from build123d import *

# Parameters (mm, degrees)
SKETCH1_W                = 110
SKETCH1_H                = 80
BOSS_EXTRUDE1_DEPTH      = 7.5
SKETCH3_W                = 110
SKETCH3_H                = 8
BOSS_EXTRUDE2_DEPTH      = 12
BOSS_EXTRUDE2_DEPTH_BACK = 12


with BuildPart() as part:
    # Sketch1 → Boss-Extrude1 (new body)
    with BuildSketch(Plane.XY):
        with Locations((0, 40)):
            Rectangle(SKETCH1_W, SKETCH1_H)
        with BuildLine():
            ThreePointArc((-27.981, 50.8), (-42.49917604, 41.099264909), (-45.905621202, 58.224621202))
            Line((-45.905621202, 58.224621202), (-38.481, 65.649242405))
            Line((-38.481, 65.649242405), (-31.056378798, 58.224621202))
            ThreePointArc((-31.056378798, 58.224621202), (-28.780264909, 54.81817604), (-27.981, 50.8))
        make_face(mode=Mode.SUBTRACT)
        with BuildLine():
            ThreePointArc((27.981, 50.8), (28.780264909, 54.81817604), (31.056378798, 58.224621202))
            Line((31.056378798, 58.224621202), (38.481, 65.649242405))
            Line((38.481, 65.649242405), (45.905621202, 58.224621202))
            ThreePointArc((45.905621202, 58.224621202), (48.181735091, 54.81817604), (48.981, 50.8))
            ThreePointArc((48.981, 50.8), (38.481, 40.3), (27.981, 50.8))
        make_face(mode=Mode.SUBTRACT)
    extrude(amount=BOSS_EXTRUDE1_DEPTH)

    # Sketch3 → Boss-Extrude2 (add, two sides)
    with BuildSketch(Plane.XY.offset(7.5)) as boss_extrude2_sk:
        with Locations((0, 4)):
            Rectangle(SKETCH3_W, SKETCH3_H)
    extrude(amount=BOSS_EXTRUDE2_DEPTH)
    extrude(boss_extrude2_sk.sketch, amount=-BOSS_EXTRUDE2_DEPTH_BACK)


solid = part.part
Input: part model. Units: mm. Frame: model coordinates. A direction names the side the tool comes from. Coordinates: 2 decimals unless noted, no trailing zeros. Loops run counter-clockwise (first coordinate to the right, second up) from the corner with the lowest first, then second, coordinate; pieces in that order, holes last.
Q1. Cut plane A-A (x = -3). Output: boundary loops of the cut face in (y, z), then the cut area to 3 significant figures.
Q2. Contact query for flat-ended pins moving along their axis: pin 1 (10 mm diameter, centred on x = -17.5, y = 64, fed in from -Z); pin 2 (3 mm diameter, centred on x = 12, y = 13, fed in from +Z); pin 3 (1 mm diameter, centred on x = 17.5, z = 13, fed in from +Y). Output: stop coordinate, or through.
Q3. Material intervals for line 1 (X direction, y = 50.8, z = 2.5); line 2 (Z direction, x = -50.5, y = 20); line 3 (Y direction, x = -46.5, z = 11), sorted ascending.
Q4. Cut plane B-B (y = 46). Output: boundary loops of the cut face in (x, z).
Q5. Cut plane D-D (y = 33.5). Output: boundary loops of the cut face in (x, z).
Q6. Cut plane C-C (x = 33). Output: boundary loops of the cut face in (y, z).
Q7. Set-up query: faces 1 (the face through (-1, 0, 8)), 2 (the face through (-1, 45, 0)), 3 (the face through (-1, 4, 19.5)), 4 (the face through (-34.82, 61.99, 3.7)), 5 (the face through (-1, 45, 7.5)). Return all of +Z, -Z, +X, -X, +Y, -Y with unobstructed straight access to the full face (end or side cutting, diameter ignored); none if empty.
Q8. Draft query along Y for faces 6 (the face through (55, 34, 4)), 7 (the face through (-1, 8, -2)), 8 (the face through (42.14, 61.99, 3.7)), 9 (the face through (34.717, 61.885, 3.698)). Return one class per face: +Y half, -Y half, draft (parallel to the pull), parting line (faces both ways), or undercut.
Working result:
1. outline: (0, -4.5) - (8, -4.5) - (8, 0) - (80, 0) - (80, 7.5) - (8, 7.5) - (8, 19.5) - (0, 19.5) - close
1. area: 732 mm2
2. pin 1: stops at z = 0
2. pin 2: stops at z = 7.5
2. pin 3: stops at y = 8
3. line 1: x = -55 to -48.98, -27.98 to 27.98, 48.98 to 55
3. line 2: z = 0 to 7.5
3. line 3: y = 0 to 8
4. outline: (-55, 0) - (-47.82, 0) - (-47.82, 7.5) - (-55, 7.5) - close; (-29.14, 0) - (29.14, 0) - (29.14, 7.5) - (-29.14, 7.5) - close; (47.82, 0) - (55, 0) - (55, 7.5) - (47.82, 7.5) - close
5. outline: (-55, 0) - (55, 0) - (55, 7.5) - (-55, 7.5) - close
6. outline: (0, -4.5) - (8, -4.5) - (8, 0) - (41.84, 0) - (41.84, 7.5) - (8, 7.5) - (8, 19.5) - (0, 19.5) - close; (60.17, 0) - (80, 0) - (80, 7.5) - (60.17, 7.5) - close
7. face 1: +Z, -Z, +X, -X, -Y
7. face 2: -Z, +X, -X, +Y
7. face 3: +Z, +X, -X, +Y, -Y
7. face 4: +Z, -Z
7. face 5: +Z, +X, -X, +Y
8. face 6: draft
8. face 7: +Y half
8. face 8: undercut
8. face 9: undercut
